Study the drawing (mm; zero at the part's minimum x, y, z) and answer. Round coordinates to 2 decimals unless told otherwise and drop trailing zeros. Write each loop counter-clockwise with the first axis right and the second up, starting at its lowest first coordinate (ties: lowest second). Pieces come first, ordered by that corner, then holes.
(1) A cutting plane is placed at C-C, the plane z = 0.75. Give the vertices of the cut face in (x, y), and give its area (3 significant figures).
(2) A cutting plane is placed at A-A, the plane y = 4.25. Give the vertices of the cut face in (x, z), and give its area (3 significant figures).
(3) Find the intervals of material crossed by probe 1 along X at (y, z) = (12.25, 2); probe 2 along Y at (x, z) = (3, 5.15); probe 3 along X at (y, z) = (10.25, 0.3), in increasing order.
(4) A cutting plane is placed at B-B, the plane x = 65. Give the vertices of the cut face in (y, z).
(5) Each of these flat-tipped pins is pushed along its axis until it touches: pin 1 Ø5.5 at (x, y) = (33.5, 1.5) entering from +Z; pin 2 Ø1 at (y, z) = (7, 1) entering from -X; pin 3 Ø0.9 at (x, y) = (66, 13.5) entering from -Z. Where does it stop, or does it pass through?
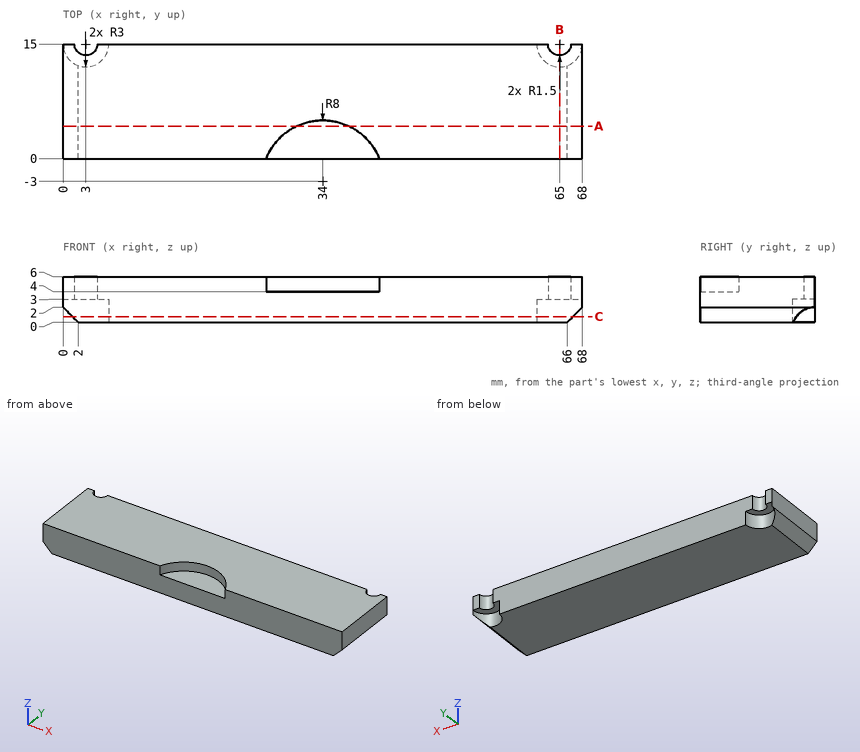
Solutions:
1. outline: (1.25, 0) - (66.75, 0) - (66.75, 12.56) arc R3 cw to (62, 15) - (6, 15) arc R3 cw to (1.25, 12.56) - close
1. area: 958 mm2
2. outline: (0, 2) - (2, 0) - (66, 0) - (68, 2) - (68, 6) - (37.38, 6) - (37.38, 4) - (30.62, 4) - (30.62, 6) - (0, 6) - close
2. area: 390 mm2
3. probe 1: x = 0 to 1.8, 4.2 to 63.8, 66.2 to 68
3. probe 2: y = 0 to 13.5
3. probe 3: x = 1.7 to 66.3
4. outline: (0, 0) - (12, 0) - (12, 3) - (13.5, 3) - (13.5, 6) - (0, 6) - close
5. pin 1: stops at z = 4
5. pin 2: stops at x = 0.5
5. pin 3: stops at z = 3
